Design review of the part shown in the three views and the two pictorial views. Dimensions are in mm from the part's minimum x, y and z. Give positions to 0.01 mm unless a question says otherwise; leave off trailing zeros. Write each loop counter-clockwise with the first axis right and the second up, starting at its lowest first coordinate (ties: lowest second). Pieces come first, ordered by that corner, then holes. Notation, with made-up numbers: M 86,15 L 93,15 A25 ccw 93,36 Z; hole C 7,70 d11. An arc over 180 degrees is marked long. Write item = value, one per line.
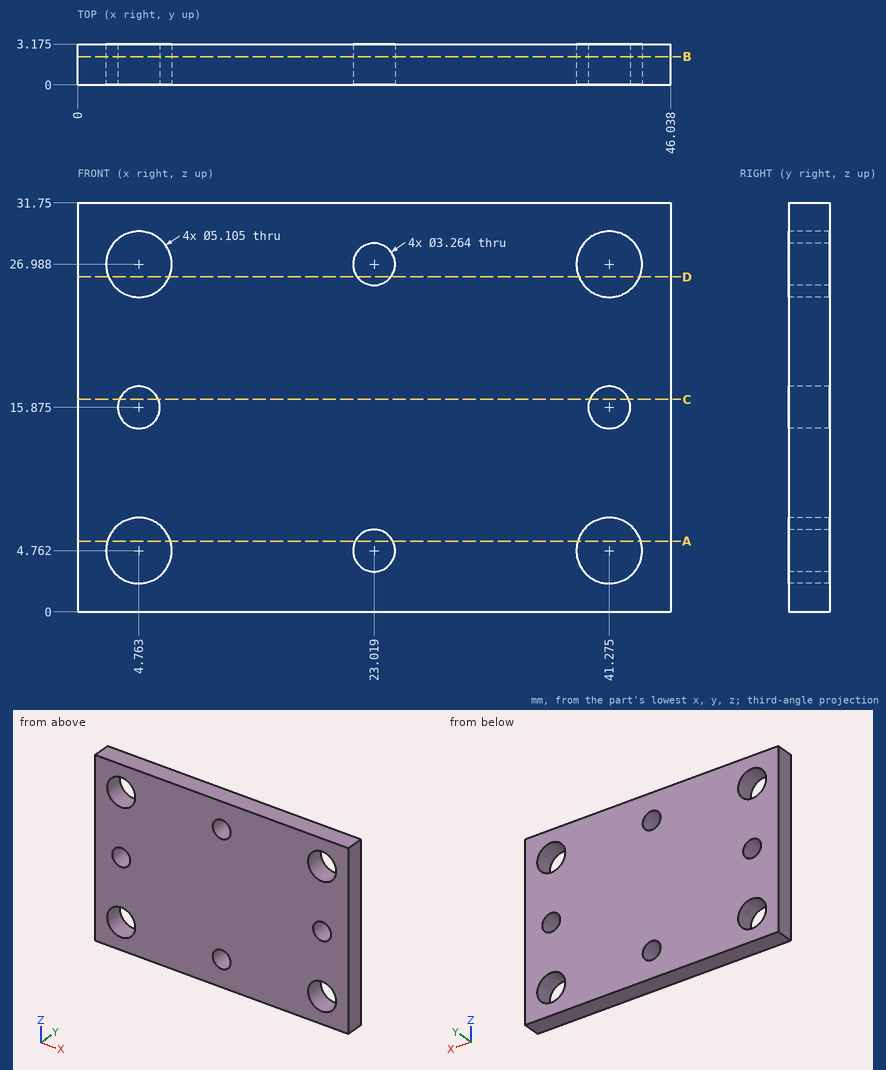
1. We need section D-D, the plane z = 26. Write out the cut boundary in (x, y) (1 decimal), then the cut area to 3 significant figures.
Responses:
outline = M 0,0 L 2.4,0 L 2.4,3.2 L 0,3.2 Z; M 7.1,0 L 21.7,0 L 21.7,3.2 L 7.1,3.2 Z; M 24.3,0 L 38.9,0 L 38.9,3.2 L 24.3,3.2 Z; M 43.6,0 L 46,0 L 46,3.2 L 43.6,3.2 Z
area = 108 mm2
2. We need section C-C, the plane z = 16.5. Write out the cut boundary in (x, y) (1 decimal), then the cut area to 3 significant figures.
Responses:
outline = M 0,0 L 3.3,0 L 3.3,3.2 L 0,3.2 Z; M 6.3,0 L 39.8,0 L 39.8,3.2 L 6.3,3.2 Z; M 42.8,0 L 46,0 L 46,3.2 L 42.8,3.2 Z
area = 127 mm2
3. We need section A-A, the plane z = 5.5. Write out the cut boundary in (x, y) (1 decimal), then the cut area to 3 significant figures.
Responses:
outline = M 0,0 L 2.3,0 L 2.3,3.2 L 0,3.2 Z; M 7.2,0 L 21.6,0 L 21.6,3.2 L 7.2,3.2 Z; M 24.5,0 L 38.8,0 L 38.8,3.2 L 24.5,3.2 Z; M 43.7,0 L 46,0 L 46,3.2 L 43.7,3.2 Z
area = 106 mm2
4. For line 1 along X through (y, z) = (2.1, 16) (1 decimal); line 2 along X through (y, z) = (0.4, 5.5) (1 decimal); line 3 along X through (y, z) = (1.5, 3) (1 decimal), list the stretches that pass through material, from the lowest coordinate up. Write a range as from..to.
Responses:
line_1 = 0..3.1, 6.4..39.6, 42.9..46
line_2 = 0..2.3, 7.2..21.6, 24.5..38.8, 43.7..46
line_3 = 0..2.9, 6.6..39.4, 43.1..46
5. We need section B-B, the plane y = 2.2. Count the separate pieces of the cut face and the enclosed holes in it, then the cut area to 3 significant figures.
Responses:
separate_pieces = 1
enclosed_holes = 8
area = 1,350 mm2
